```python
from build123d import *

# Parameters (mm, degrees)
SZKIC1_R                    = 1.55
DODANIE_WYCI_GNI_CIE1_DEPTH = 10


with BuildPart() as part:
    # Szkic1 → Dodanie-wyciągnięcie1 (new body)
    with BuildSketch(Plane.XY):
        with BuildLine():
            Line((-179.126801066, 83.617157096), (-183.434880274, 83.617157096))
            ThreePointArc((-183.434880274, 83.617157096), (-187.377274513, 80.293565011), (-184.768213607, 75.84592093))
            ThreePointArc((-184.768213607, 75.84592093), (-183.801887112, 75.115003385), (-183.434880274, 73.960302847))
            Line((-183.434880274, 73.960302847), (-183.434880274, 57.530770571))
            ThreePointArc((-183.434880274, 57.530770571), (-175.434880274, 49.530770571), (-167.434880274, 57.530770571))
            Line((-167.434880274, 57.530770571), (-167.434880274, 73.777889147))
            ThreePointArc((-167.434880274, 73.777889147), (-171.51222692, 80.799152225), (-179.126801066, 83.617157096))
        make_face()
        with Locations((-175.434880274, 57.530770571)):
            Circle(SZKIC1_R, mode=Mode.SUBTRACT)
        with Locations((-175.434880274, 71.530770571)):
            Circle(SZKIC1_R, mode=Mode.SUBTRACT)
    extrude(amount=DODANIE_WYCI_GNI_CIE1_DEPTH)


solid = part.part
```
The listing builds one solid part. Answer for the finished solid, in the listing's coordinates (mm). A direction names the side the tool comes from. Give positions to 0.01 mm unless a question says otherwise; leave off trailing zeros. Write each loop counter-clockwise with the first axis right and the second up, starting at its lowest first coordinate (ties: lowest second). Pieces come first, ordered by that corner, then holes. Notation, with made-up numbers: (-25.75, -33) - (-13.75, -33) arc R5 cw to (-13.75, -28) - close; hole circle Ø2 at (47.25, 48). An arc over 180 degrees is marked (long way). Use one line per item in the form item = value. Start each with the question number.
1) Find section C-C on y = 57. Determine the outline of the cut face in (x, z).
2) Find section B-B on z = 3. Determine the outline of the cut face in (x, y), plus the area to 3 significant figures.
3) The mould has two halves that part along X. Classify faces 1 (the face through (-187.363, 80.371, 4.93)), 2 (the face through (-176.983, 57.599, 4.93)), 3 (the face through (-175.611, 49.533, 4.93)): pulls with the +X half, pulls with the -X half, needs draft (parallel to the pull), parting line crosses it, or undercut.
4) Find section D-D on y = 75.5. Determine the outline of the cut face in (x, z), plus the area to 3 significant figures.
5) Consider line 1 along X through (y, z) = (64, 1.75); line 2 along Y through (x, z) = (-175.75, 7.75); line 3 along Y through (x, z) = (-174.25, 2.75). Determine where each line is inside the solid, lowest interval first. Write a range as from..to.
6) Flat-ended cylindrical pins translate along their axes: pin 1 Ø1.5 at (x, z) = (-174, 1.5) entering from +Y; pin 2 Ø3 at (y, z) = (65.5, 4.5) entering from -X; pin 3 Ø6 at (x, z) = (-175.5, 4.5) entering from +Y. Find the tip coordinate at first contact, or state that the pin passes through.
7) A tool of negligible diameter and unlimited length cuts with its end or side. For faces 4 (the face through (-183.435, 66, 5)), 5 (the face through (-181, 83.617, 5)), from which of +Z, -Z, +X, -X, +Y, -Y can it reach the whole face along a straight path? Write none if from no direction.
8) Find section A-A on x = -176. Determine the outline of the cut face in (y, z), plus the area to 3 significant figures.
Geometry results:
q1.outline = (-183.42, 0) - (-176.89, 0) - (-176.89, 10) - (-183.42, 10) - close; (-173.98, 0) - (-167.45, 0) - (-167.45, 10) - (-173.98, 10) - close
q2.outline = (-184.77, 75.85) arc R2 cw to (-183.43, 73.96) - (-183.43, 57.53) arc R8 ccw to (-167.43, 57.53) - (-167.43, 73.78) arc R12 ccw to (-179.13, 83.62) - (-183.43, 83.62) arc R4 ccw to start; hole circle Ø3.1 at (-175.43, 57.53); hole circle Ø3.1 at (-175.43, 71.53)
q2.area = 500 mm2
q3.face_1 = pulls with the -X half
q3.face_2 = undercut
q3.face_3 = parting line crosses it
q4.outline = (-184.16, 0) - (-167.88, 0) - (-167.88, 10) - (-184.16, 10) - close
q4.area = 163 mm2
q5.line_1 = -183.43..-167.43
q5.line_2 = 49.54..56.01, 59.05..70.01, 73.05..83.1
q5.line_3 = 49.62..56.53, 58.53..70.53, 72.53..82.53
q6.pin_1 = 82.75
q6.pin_2 = -183.43
q6.pin_3 = 83.59
q7.face_4 = +Z, -Z, -X, -Y
q7.face_5 = +Z, -Z, +X, -X, +Y
q8.outline = (49.55, 0) - (56.09, 0) - (56.09, 10) - (49.55, 10) - close; (58.97, 0) - (70.09, 0) - (70.09, 10) - (58.97, 10) - close; (72.97, 0) - (83.17, 0) - (83.17, 10) - (72.97, 10) - close
q8.area = 278 mm2
